Autodesk Inventor part; units mm, degrees
ref_plane "YZ Plane" through (0, 0, 0) normal (1, 0, 0) x (0, 1, 0)
ref_plane "XZ Plane" through (0, 0, 0) normal (0, 1, 0) x (-1, 0, 0)
ref_plane "XY Plane" through (0, 0, 0) normal (0, 0, 1) x (1, 0, 0)
sketch "スケッチ1" plane through (0, 0, 0) normal (1, 0, 0) x (0, 1, 0)
  circle A0 centre (0, 0) radius 6.25
  line L0 (0, 13) -> (-24, 13)
  line L1 (-24, 13) -> (-24, -13)
  line L2 (-24, -13) -> (0, -13)
  line L3 (0, -13) -> (0, 13) construction
  line L4 (0, 13) -> (13, 13)
  line L5 (13, 13) -> (13, -13)
  line L6 (13, -13) -> (0, -13)
  line L7 (0, -13) -> (0, 13)
  dimension "d0" = 12.5
  dimension "d1" = 24
  dimension "d2" = 26
  dimension "d3" = 13
extrude "プレート1" add sketch "スケッチ1" along normal blind 1.5 contours A0 L7 L4 L5 L6 | A0 L7 L2 L1 L0
sketch "スケッチ2" plane through (1.5, 11.5, -13) normal (0, 1, 0) x (-1, 0, 0)
  line L0 (0, 26) -> (0, 0)
  line L1 (0, 0) -> (10, 0)
  line L2 (10, 0) -> (10, 26)
  line L3 (10, 26) -> (0, 26)
edge flange "フランジ1" height 10 angle 90 thickness 1.5 bend radius 1.5 thickness toward (0, 1, 0) relief tear relief width 1.5 relief depth 0.75 edges at (0, 13, 0) wall of the first edge with corners at (1.5, 11.5, 13) (1.5, 11.5, -13) (-8.5, 11.5, -13) (-8.5, 11.5, 13)
bend "曲げ1"
corner "コーナー1"
sketch "スケッチ3" plane through (1.5, 0, 0) normal (1, 0, 0) x (0, 0, -1)
  circle A0 centre (10.5, 0) radius 1
  circle A1 centre (-10.5, 0) radius 1
  circle A2 centre (-10.5, -21) radius 1
  circle A3 centre (10.5, -21) radius 1
  point P0 (0, 0)
extrude "切り取り1" cut sketch "スケッチ3" against normal blind 1.5
sketch "スケッチ4" plane through (1.5, 0, 0) normal (1, 0, 0) x (0, 0, -1)
  circle A0 centre (-10.5, -21) radius 1
  circle A1 centre (10.5, 0) radius 1
  circle A2 centre (-10.5, 0) radius 1
  circle A3 centre (10.5, -21) radius 1
  line L0 (13, 10) -> (-13, 10)
  line L1 (-13, -24) -> (-13, 10)
  line L2 (13, -24) -> (-13, -24)
  line L3 (13, 10) -> (13, -24)
  circle A4 centre (0, 0) radius 6.25
  line L4 (-10.5, 0) -> (10.5, 0)
  line L5 (10.5, 0) -> (10.5, -21)
  line L6 (10.5, -21) -> (-10.5, -21)
  line L7 (-10.5, -21) -> (-10.5, 0)
  line L8 (-10.5, -2) -> (10.5, -2)
  line L9 (10.5, -2) -> (10.5, -19)
  line L10 (10.5, -19) -> (-10.5, -19)
  line L11 (-10.5, -19) -> (-10.5, -2)
  dimension "d17" = 2
  dimension "d18" = 2
extrude "切り取り2" cut sketch "スケッチ4" against normal blind 1.5 contours L7 L8 A4 L5 L10 | L8 A4
sketch "スケッチ5" plane through (-8.5, 13, 13) normal (0, 1, 0) x (1, 0, 0)
  circle A0 centre (2, 21) radius 0.8
  circle A1 centre (2, 5) radius 0.8
  line L0 (0, 0) -> (0, 26)
  line L1 (0, 26) -> (7, 26)
  line L2 (7, 0) -> (0, 0)
  point P0 (8.5, 13)
  dimension "d21" = 1.6
  dimension "d23" = 2
  dimension "d24" = 5
  dimension "d25" = 5
extrude "切り取り3" cut sketch "スケッチ5" against normal blind 1.5
fillet "フィレット1" radius 3 10 edges at (-8.5, 12.25, -13) (-8.5, 12.25, 13) (0.75, -2, 5.9214) (0.75, -2, -5.9214) (0.75, -2, -10.5) (0.75, -2, 10.5) (0.75, -24, -13) (0.75, -24, 13) (0.75, -19, -10.5) (0.75, -19, 10.5)
equation "\"d15\" = Thickness"
equation "\"d18\" = d17"
equation "\"d19\" = Thickness"
equation "\"d25\" = d24"
equation "\"d26\" = Thickness"
equation "\"d4\" = Thickness"
equation "\"d5\" = BendReliefWidth"
equation "\"d6\" = BendReliefDepth"
equation "\"d7\" = MinimumRemnant"
equation "\"d8\" = TransitionRadius"
equation "\"d11\" = BendRadius"
equation "\"d12\" = CornerReliefSize"
equation "\"d13\" = GapSize"
equation "\"d14\" = JacobiRadiusSize"
equation "\"BendRadius\" = Thickness"
equation "\"BendReliefWidth\" = Thickness"
equation "\"BendReliefDepth\" = 0.5 * Thickness"
equation "\"CornerReliefSize\" = 4 * Thickness"
equation "\"MinimumRemnant\" = 2 * Thickness"
equation "\"TransitionRadius\" = BendRadius"
equation "\"JacobiRadiusSize\" = BendRadius"
equation "\"GapSize\" = Thickness"
properties part number "neck_joint"
Part model, mm, in its own coordinate system. A direction names the side the tool comes from. Coordinates: 2 decimals unless noted, no trailing zeros. Write each loop counter-clockwise with the first axis right and the second up, starting at its lowest first coordinate (ties: lowest second). Pieces come first, ordered by that corner, then holes.
Item 1: Probe line 1 (X direction, y = 12.6, z = 8); line 2 (Z direction, x = -6.5, y = 12.55); line 3 (X direction, y = 4, z = -6). List the from-to ranges inside material, lowest first.
Item 2: Slice it at C-C (y = 0). Write the cut outline in (x, z), and give its area (3 significant figures).
Item 3: Mould opens along Y. For faces 3 (the face through (0.74, -23.1, -12.14)), 4 (the face through (1, -3, 13)), 5 (the face through (1, -10, 10.5)) say: released by +Y, released by -Y, zero draft, split by the parting line, or undercut.
Item 4: Which spindle directions (+Z, -Z, +X, -X, +Y, -Y) get a long thin tool onto all of the face, cutting with end or side? Do faces 1 (the face through (-7.3, 12.3, 8)), 2 (the face through (0.76, -18.1, 9.64)). Say none if no direction does.
Item 5: Slice it at B-B (z = 5.75). Write the cut outline in (x, y), and give its area (3 significant figures).
Item 6: Slice it at D-D (x = -4.75). Write the cut outline in (y, z), and give its area (3 significant figures).
Item 7: Slice it at A-A (y = -11). Write the cut outline in (x, z), and give its area (3 significant figures).
Item 8: Pin check, flat tips, straight feed: pin 1 (1.6 mm diameter, centred on x = 0.5, z = 1, fed in from +Y); pin 2 (1.8 mm diameter, centred on y = 0, z = 10.5, fed in from -X); pin 3 (3 mm diameter, centred on x = -4.5, z = 8.5, fed in from -Y). Stop position of each tip, or through.
Results found:
1. line 1: x = -8.5 to -7.3, -5.7 to 0
1. line 2: z = -12.83 to -8.8, -7.2 to 7.2, 8.8 to 12.83
1. line 3: x = 0 to 1.5
2. outline: (0, -13) - (1.5, -13) - (1.5, -11.5) - (0, -11.5) - close; (0, -9.5) - (1.5, -9.5) - (1.5, -6.37) - (0, -6.37) - close; (0, 6.37) - (1.5, 6.37) - (1.5, 9.5) - (0, 9.5) - close; (0, 11.5) - (1.5, 11.5) - (1.5, 13) - (0, 13) - close
2. area: 13.9 mm2
3. face 3: released by -Y
3. face 4: zero draft
3. face 5: undercut
4. face 1: +Y, -Y
4. face 2: +X, -X
5. outline: (-8.5, 11.5) - (-1.5, 11.5) arc R1.5 cw to (0, 10) - (0, 2.45) - (1.5, 2.45) - (1.5, 10) arc R3 ccw to (-1.5, 13) - (-8.5, 13) - close; (0, -24) - (1.5, -24) - (1.5, -19) - (0, -19) - close
5. area: 34.6 mm2
6. outline: (11.5, -13) - (13, -13) - (13, 13) - (11.5, 13) - close
6. area: 39.0 mm2
7. outline: (0, -13) - (1.5, -13) - (1.5, -10.5) - (0, -10.5) - close; (0, 10.5) - (1.5, 10.5) - (1.5, 13) - (0, 13) - close
7. area: 7.50 mm2
8. pin 1: stops at y = 12.75
8. pin 2: passes through
8. pin 3: stops at y = 11.5
